Check sheet for the modelled part. Datum: model origin and axes. Units: mm. A direction names the side the tool comes from. Coordinates: 2 decimals unless noted, no trailing zeros. Loops run counter-clockwise (first coordinate to the right, second up) from the corner with the lowest first, then second, coordinate; pieces in that order, holes last. Notation, with made-up numbers: (54, -4.75) -> (72, -4.75) arc R23 ccw to (72, 8.25) -> close; hole circle Ø4 at (-29.75, 57). An arc over 180 degrees is marked (long way). Use CSV: the item, a comma, the result in double quotes.
```python
from build123d import *

# Parameters (mm, degrees)
F1_DEPTH = 5
F2_R     = 4.49999
F3_R     = 0.5


# Not quite as in the source:
# - a fillet or chamfer is up to 0.001 mm smaller than in the source, because OpenCascade refuses the exact size


with BuildPart() as f1:
    # F0 (on Top) → F1 (new body)
    with BuildSketch(Plane.XY):
        Polygon((4.5, -14.5), (4.5, 14.5), (0, 14.5), (-4.5, 14.5), (-4.5, -14.5), (0, -14.5), align=None)
        Polygon((2.2, -12.2), (0, -12.2), (-2.2, -12.2), (-2.2, -7.8), (2.2, -7.8), align=None, mode=Mode.SUBTRACT)
        Polygon((-2.2, 12.2), (0, 12.2), (2.2, 12.2), (2.2, 7.8), (-2.2, 7.8), align=None, mode=Mode.SUBTRACT)
    extrude(amount=F1_DEPTH)

    # F2 (radius 4.5 in the source; OpenCascade refuses exactly that, so slightly less here)
    f2_edges = [f1.edges().sort_by_distance(p)[0] for p in [
        (-4.5, 14.5, 2.5),
        (4.5, 14.5, 2.5),
        (4.5, -14.5, 2.5),
        (-4.5, -14.5, 2.5),
    ]]
    fillet(f2_edges, radius=F2_R)

    # F3
    f3_edges = [f1.edges().sort_by_distance(p)[0] for p in [
        (-4.5, 0, 5),
        (-4.5, 0, 0),
    ]]
    fillet(f3_edges, radius=F3_R)


solid = f1.part
```
1) Cross-section at B-B on y = 9. Record the boundary of the cut face in (x, z).
Answer below:
outline,"(-4.5, 0.5) arc R0.5 ccw to (-4, 0) -> (-2.2, 0) -> (-2.2, 5) -> (-4, 5) arc R0.5 ccw to (-4.5, 4.5) -> close; (2.2, 0) -> (4, 0) arc R0.5 ccw to (4.5, 0.5) -> (4.5, 4.5) arc R0.5 ccw to (4, 5) -> (2.2, 5) -> close"
2) Access from +Z, -Z, +X, -X, +Y, -Y to the whole of each face (thin tool, end or side, straight path). Record for faces 4 (the flat face through (-2.2, 10, 2)), 5 (the cylindrical face through (3.217, 13.147, 2.528)).
Answer below:
face 4,"+Z, -Z"
face 5,"+Z, -Z, +X, +Y"
3) Thickness scan on line 1 along Y through (x, z) = (0.25, 3.1); line 2 along Y through (x, z) = (1.75, 4.3); line 3 along X through (y, z) = (-9.25, 2.5). Record the ranges inside material, lowest first. Write a range as from..to.
Answer below:
line 1,"y = -14.49..-12.2, -7.8..7.8, 12.2..14.49"
line 2,"y = -14.15..-12.2, -7.8..7.8, 12.2..14.15"
line 3,"x = -4.5..-2.2, 2.2..4.5"
4) Draft check along X on faces 1 (the cylindrical face through (3.217, -13.147, 2.528)), 2 (the cylindrical face through (-3.217, -13.147, 2.528)), 3 (the flat face through (0, -7.8, 2)). Enter one of: released by +X, released by -X, zero draft, split by the parting line, or undercut.
Answer below:
face 1,"released by +X"
face 2,"released by -X"
face 3,"undercut"
5) Go/stop test with flat-tipped pins: pin 1 Ø3 at (x, z) = (3, 2) entering from -Y; pin 2 Ø1.3 at (x, z) = (1, 2.5) entering from -Y; pin 3 Ø1.5 at (x, z) = (-1, 4) entering from +Y. Record where each tip stops, or that it passes through.
Answer below:
pin 1,"stops at y = -14.24"
pin 2,"stops at y = -14.49"
pin 3,"stops at y = 14.49"
6) Cross-section at A-A on z = 2.9. Give the number of separate pieces and of enclosed holes in the cut face, and give its area (3 significant figures).
Answer below:
separate pieces,"1"
enclosed holes,"2"
area,"205 mm²"
